The model under review builds one solid part; all positions refer to its coordinate system, in mm. Face numbers are marked on the shaded views. A direction names the side the tool comes from. Give positions to 0.01 mm unless a question says otherwise; leave off trailing zeros. Order: outer loops, then holes, each group sorted by start corner. A loop starts at its lowest first (then second) coordinate and runs counter-clockwise, first axis right, second up. Notation, with made-up numbers: (-31.75, 87.25) - (-5.75, 87.25) arc R19 ccw to (-5.75, 91.25) - close; hole circle Ø8 at (44, 41.25). An arc over 180 degrees is marked (long way). Use CSV: the item, a comma, the result in double quotes. Start each with the question number.
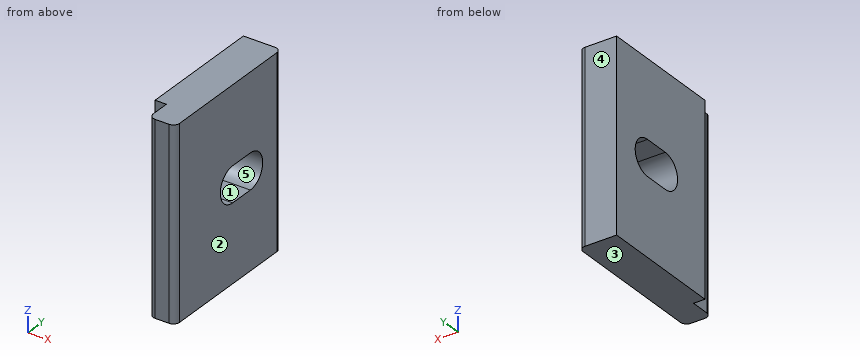
```python
from build123d import *

# Parameters (mm, degrees)
PAD_DEPTH    = 15
POCKET_DEPTH = 3.001


with BuildPart() as part:
    # Sketch → Pad (new body)
    with BuildSketch(Plane.XY):
        with BuildLine():
            Line((0, 10), (0, 0))
            Line((0, 0), (0.9, 0))
            Line((0.9, 0), (0.9, -1.5))
            ThreePointArc((0.9, -1.5), (1.046447, -1.853553), (1.4, -2))
            Line((1.4, -2), (2.5, -2))
            ThreePointArc((2.5, -2), (2.853553, -1.853553), (3, -1.5))
            Line((3, -1.5), (3, 9.5))
            ThreePointArc((3, 9.5), (2.853553, 9.853553), (2.5, 10))
            Line((2.5, 10), (0, 10))
        make_face()
    extrude(amount=PAD_DEPTH)

    # Sketch001 → Pocket (cut, through all)
    with BuildSketch(Plane.YZ.offset(3)):
        with BuildLine():
            ThreePointArc((4.5, 8.9), (3.1, 7.5), (4.5, 6.1))
            Line((4.5, 6.1), (6.5, 6.1))
            ThreePointArc((6.5, 6.1), (7.9, 7.5), (6.5, 8.9))
            Line((4.5, 8.9), (6.5, 8.9))
        make_face()
    extrude(amount=-POCKET_DEPTH, mode=Mode.SUBTRACT)


solid = part.part
```
1. Clearance check with a flat-ended pin moving along its axis: pin 1 (1.2 mm diameter, centred on y = -1, z = 11, fed in from -X). State where the tip first meets the part, or that it passes through.
2. To check wall thickness, follow L1, parallel to Z at x = 0.8, y = 6.5; L2, parallel to X at y = -0.25, z = 12; L3, parallel to Y at x = 0.6, z = 11.5. State the ranges of each line that lie inside material, in increasing order. Write a range as [from, to].
3. Tool access review of the marked faces 1 and 2: name each direction out of +Z, -Z, +X, -X, +Y, -Y from which nothing blocks a thin tool from reaching the whole face with its end or side.
4. Mouldability with a two-part tool opening along Z and no side actions: class the marked faces 3, 4 and 5 as pulls with the +Z half, pulls with the -Z half, needs draft (parallel to the pull), parting line crosses it, or undercut.
5. Consider section B-B (x = 1.6). Give the boundary of the cut face in (y, z), and give its area (3 significant figures).
6. Consider section A-A (z = 7.5). Give the boundary of the cut face in (x, y), and give its area (3 significant figures).
7. Consider section D-D (z = 9.5). Give the boundary of the cut face in (x, y).
8. Consider section C-C (y = 6.25). Give the boundary of the cut face in (x, z).
Answers follow:
1,pin 1,"stops at x = 0.9"
2,L1,"z = [0, 6.1], [8.9, 15]"
2,L2,"x = [0.9, 3]"
2,L3,"y = [0, 10]"
3,face 1,"+X, -X"
3,face 2,"+Z, -Z, +X, +Y, -Y"
4,face 3,"pulls with the -Z half"
4,face 4,"needs draft"
4,face 5,"undercut"
5,outline,"(-2, 0) - (10, 0) - (10, 15) - (-2, 15) - close; hole (4.5, 6.1) - (6.5, 6.1) arc R1.4 ccw to (6.5, 8.9) - (4.5, 8.9) arc R1.4 ccw to start"
5,area,"168 mm^2"
6,outline,"(0, 0) - (0.9, 0) - (0.9, -1.5) arc R0.5 ccw to (1.4, -2) - (2.5, -2) arc R0.5 ccw to (3, -1.5) - (3, 3.1) - (0, 3.1) - close; (0, 7.9) - (3, 7.9) - (3, 9.5) arc R0.5 ccw to (2.5, 10) - (0, 10) - close"
6,area,"19.6 mm^2"
7,outline,"(0, 0) - (0.9, 0) - (0.9, -1.5) arc R0.5 ccw to (1.4, -2) - (2.5, -2) arc R0.5 ccw to (3, -1.5) - (3, 9.5) arc R0.5 ccw to (2.5, 10) - (0, 10) - close"
8,outline,"(0, 0) - (3, 0) - (3, 6.1) - (0, 6.1) - close; (0, 8.9) - (3, 8.9) - (3, 15) - (0, 15) - close"
